The listing builds one solid part. Answer for the finished solid, in the listing's coordinates (mm). A direction names the side the tool comes from. Give positions to 0.01 mm unless a question says otherwise; leave off trailing zeros. Order: outer loops, then holes, each group sorted by start corner. A loop starts at its lowest first (then second) coordinate and runs counter-clockwise, first axis right, second up. Notation, with made-up numbers: (3.25, -12.75) - (38.25, -12.75) arc R28 ccw to (38.25, 14.25) - close; hole circle Ø11 at (4, 3). An arc over 180 degrees is marked (long way). Answer in a Markdown table with one row per item.
from build123d import *

# Parameters (mm, degrees)
BOSS_EXTRUDE1_DEPTH = 304.8
SKETCH11_R          = 2.05
CUT_EXTRUDE1_DEPTH  = 50.8


with BuildPart() as part:
    # Sketch2 → Boss-Extrude1 (new, symmetric)
    with BuildSketch(Plane.XY):
        with BuildLine():
            Line((-12.7, -12.7), (12.7, -12.7))
            Line((12.7, -12.7), (12.7, 12.7))
            Line((12.7, 12.7), (11.1125, 12.7))
            ThreePointArc((11.1125, 12.7), (9.989967985, 12.235032015), (9.525, 11.1125))
            Line((9.525, 11.1125), (9.525, -6.35))
            ThreePointArc((9.525, -6.35), (8.59506403, -8.59506403), (6.35, -9.525))
            Line((6.35, -9.525), (-11.1125, -9.525))
            ThreePointArc((-11.1125, -9.525), (-12.235032015, -9.989967985), (-12.7, -11.1125))
            Line((-12.7, -11.1125), (-12.7, -12.7))
        make_face()
    extrude(amount=BOSS_EXTRUDE1_DEPTH, both=True)

    # Sketch11 → Cut-Extrude1 (cut)
    with BuildSketch(Plane(origin=(12.7, 0, 0), x_dir=(0, 0, -1), z_dir=(1, 0, 0))):
        with Locations(Location((288.925, 0, 0), (0, 0, 90))):
            Circle(SKETCH11_R)
        with Locations(Location((282.575, 6.35, 0), (0, 0, 90))):
            Circle(SKETCH11_R)
        with Locations(Location((266.7, 0, 0), (0, 0, 90))):
            Circle(SKETCH11_R)
        with Locations(Location((228.6, 0, 0), (0, 0, 90))):
            Circle(SKETCH11_R)
        with Locations(Location((190.5, 0, 0), (0, 0, 90))):
            Circle(SKETCH11_R)
        with Locations(Location((152.4, 0, 0), (0, 0, 90))):
            Circle(SKETCH11_R)
        with Locations(Location((114.3, 0, 0), (0, 0, 90))):
            Circle(SKETCH11_R)
        with Locations(Location((76.2, 0, 0), (0, 0, 90))):
            Circle(SKETCH11_R)
        with Locations(Location((38.1, 0, 0), (0, 0, 90))):
            Circle(SKETCH11_R)
        with Locations(Location((0, 0, 0), (0, 0, 90))):
            Circle(SKETCH11_R)
        with Locations(Location((-38.1, 0, 0), (0, 0, 90))):
            Circle(SKETCH11_R)
        with Locations(Location((-76.2, 0, 0), (0, 0, 90))):
            Circle(SKETCH11_R)
        with Locations(Location((-114.3, 0, 0), (0, 0, 90))):
            Circle(SKETCH11_R)
        with Locations(Location((-152.4, 0, 0), (0, 0, 90))):
            Circle(SKETCH11_R)
        with Locations(Location((-190.5, 0, 0), (0, 0, 90))):
            Circle(SKETCH11_R)
        with Locations(Location((-228.6, 0, 0), (0, 0, 90))):
            Circle(SKETCH11_R)
        with Locations(Location((-266.7, 0, 0), (0, 0, 90))):
            Circle(SKETCH11_R)
        with Locations(Location((-282.575, 6.35, 0), (0, 0, 90))):
            Circle(SKETCH11_R)
        with Locations(Location((-288.925, 0, 0), (0, 0, 90))):
            Circle(SKETCH11_R)
    extrude(amount=-CUT_EXTRUDE1_DEPTH, mode=Mode.SUBTRACT)


solid = part.part
Item 1: Each of these flat-tipped pins is pushed along its axis until it touches: P1, Ø3.5, axis at y = 0, z = 228.6, coming from the +X side; P2, Ø4, axis at x = 1, z = 170, coming from the +Y side (3 decimals); P3, Ø6.5, axis at y = 6.35, z = 282.575, coming from the -X side (3 decimals). Where does it stop, or does it pass through?
Answer block:
| item | result |
|---|---|
| P1 | through |
| P2 | y = -9.525 |
| P3 | x = 9.525 |
Item 2: Consider line 1 (Y direction, x = 11.1, z = -228.6); line 2 (Y direction, x = -10.25, z = -29) (3 decimals); line 3 (X direction, y = 10.5, z = -124.5) (3 decimals). Determine where each line is inside the solid, lowest interval first.
Answer block:
| item | result |
|---|---|
| line 1 | -12.7 to -2.05, 2.05 to 12.7 |
| line 2 | -12.7 to -9.525 |
| line 3 | 9.525 to 12.7 |
Item 3: Find section B-B on x = -2.75. Write down the section's boundary in (y, z) (3 decimals), then the cut area to 3 significant figures.
Answer block:
| item | result |
|---|---|
| outline | (-12.7, -304.8) - (-9.525, -304.8) - (-9.525, 304.8) - (-12.7, 304.8) - close |
| area | 1,940 mm² |
Item 4: Which of the six approach directions +Z, -Z, +X, -X, +Y, -Y give full straight-line access (tool end or side, diameter ignored) to faces 1 (the face through (6, -10, -304.8)), 2 (the face through (9.525, 3, 4))?
Answer block:
| item | result |
|---|---|
| face 1 | -Z, +X, -X, +Y, -Y |
| face 2 | +Z, -Z, -X, +Y |
